Read the model definition and answer for the solid it produces. Units are mm, in the model's axes. Face numbers are marked on the shaded views. A direction names the side the tool comes from. Give positions to 0.01 mm unless a question says otherwise; leave off trailing zeros. Order: outer loops, then holes, each group sorted by start corner. A loop starts at its lowest first (then second) coordinate and runs counter-clockwise, first axis right, second up. Notation, with made-up numbers: (60, -25.75) - (101, -25.75) arc R26 cw to (101, 3.25) - close; hole circle Ø9 at (-3, -22.75). An arc over 180 degrees is marked (long way). Write item = value, one per line.
```python
from build123d import *

# Parameters (mm, degrees)
F0_W     = 1100
F0_H     = 1100
F1_DEPTH = 150
F2_W     = 100
F2_H     = 900
F3_DEPTH = 150


with BuildPart() as f1:
    # F0 (on Top) → F1 (new body)
    with BuildSketch(Plane.XY):
        Rectangle(F0_W, F0_H)
    extrude(amount=F1_DEPTH)

    # F2 (on face) → F3 (cut)
    with BuildSketch(Plane.XY.offset(150)):
        with Locations((-400, 0)):
            Rectangle(F2_W, F2_H)
        with Locations((-240, 0)):
            Rectangle(F2_W, F2_H)
        with Locations((-80, 0)):
            Rectangle(F2_W, F2_H)
        with Locations((80, 0)):
            Rectangle(F2_W, F2_H)
        with Locations((240, 0)):
            Rectangle(F2_W, F2_H)
        with Locations((400, 0)):
            Rectangle(F2_W, F2_H)
    extrude(amount=-F3_DEPTH, mode=Mode.SUBTRACT)


solid = f1.part
```
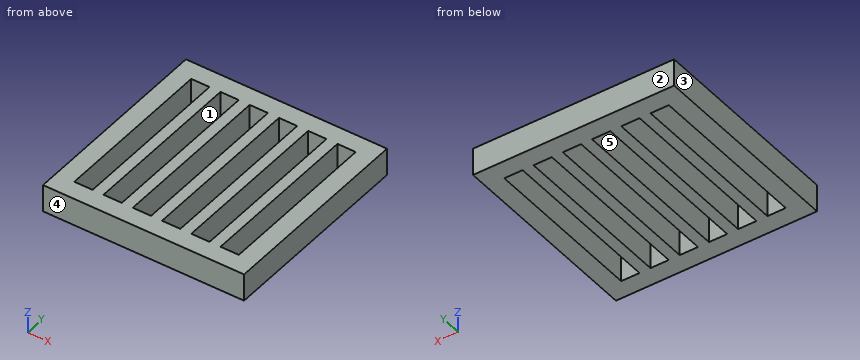
1. Section B-B (y = -151) is taken. Determine the outline of the cut face in (x, z).
Recorded:
outline = (-550, 0) - (-450, 0) - (-450, 150) - (-550, 150) - close; (-350, 0) - (-290, 0) - (-290, 150) - (-350, 150) - close; (-190, 0) - (-130, 0) - (-130, 150) - (-190, 150) - close; (-30, 0) - (30, 0) - (30, 150) - (-30, 150) - close; (130, 0) - (190, 0) - (190, 150) - (130, 150) - close; (290, 0) - (350, 0) - (350, 150) - (290, 150) - close; (450, 0) - (550, 0) - (550, 150) - (450, 150) - close
2. Section C-C (x = 75) is taken. Determine the outline of the cut face in (y, z).
Recorded:
outline = (-550, 0) - (-450, 0) - (-450, 150) - (-550, 150) - close; (450, 0) - (550, 0) - (550, 150) - (450, 150) - close
3. Determine the mould class of the marked faces 1, 2 and 3 for opening direction Y: +Y half, -Y half, draft (parallel to the pull), parting line (faces both ways), or undercut.
Recorded:
face_1 = undercut
face_2 = +Y half
face_3 = draft
4. A straight line is drawn through the part: L1, parallel to Y at x = 228, z = 57. Find the intervals that lie inside material, in ascending order. Write a range as [from, to].
Recorded:
L1 = [-550, -450], [450, 550]
5. For the marked faces 4 and 5, determine the directions among +Z, -Z, +X, -X, +Y, -Y from which every point of the face is accessible in a straight line to the end or side of a thin tool.
Recorded:
face_4 = +Z, -Z, +X, -X, -Y
face_5 = +Z, -Z
6. Section A-A (z = 127) is taken. Determine the outline of the cut face in (x, y).
Recorded:
outline = (-550, -550) - (550, -550) - (550, 550) - (-550, 550) - close; hole (-450, -450) - (-350, -450) - (-350, 450) - (-450, 450) - close; hole (-290, -450) - (-190, -450) - (-190, 450) - (-290, 450) - close; hole (-130, -450) - (-30, -450) - (-30, 450) - (-130, 450) - close; hole (30, -450) - (130, -450) - (130, 450) - (30, 450) - close; hole (190, -450) - (290, -450) - (290, 450) - (190, 450) - close; hole (350, -450) - (450, -450) - (450, 450) - (350, 450) - close
